Here's how the part is built. I have some questions about the finished solid (model axes, mm). Face numbers are marked on the shaded views. A direction names the side the tool comes from. Coordinates: 2 decimals unless noted, no trailing zeros. Order: outer loops, then holes, each group sorted by start corner. A loop starts at its lowest first (then second) coordinate and runs counter-clockwise, first axis right, second up. Notation, with made-up numbers: (13, 58) - (59, 58) arc R27 cw to (59, 80) - close; hole circle Ø4 at (65, 51). An arc over 180 degrees is marked (long way). Use one line per item in the form item = value. Start each with the question number.
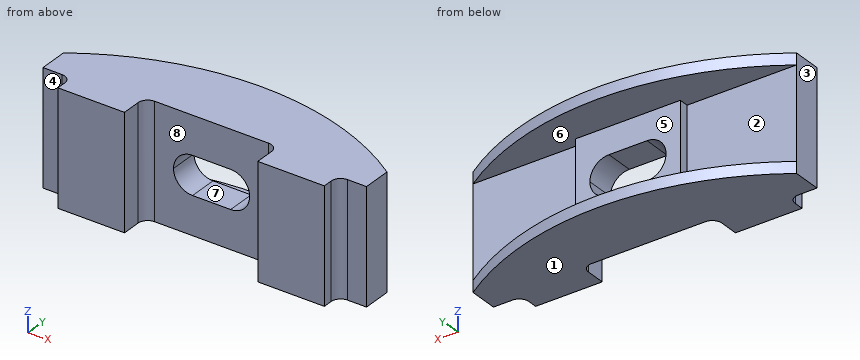
from build123d import *

# Parameters (mm, degrees)
F0_W      = 170
F0_H      = 60
F1_DEPTH  = 30
F2_W      = 70
F2_H      = 30
F3_DEPTH  = 59.69157
F4_R      = 5
F6_DEPTH  = 60.001
F7_W      = 57.5
F7_H      = 5
F8_DEPTH  = 60.001
F10_DEPTH = 6
F13_DEPTH = 30.001


with BuildPart() as f1:
    # F0 (on Front) → F1 (new body)
    with BuildSketch(Plane.XZ):
        Rectangle(F0_W, F0_H)
    extrude(amount=F1_DEPTH)

    # F2 (on Top) → F3 (cut, symmetric)
    with BuildSketch(Plane.XY):
        with Locations((0, -30)):
            Rectangle(F2_W, F2_H)
    extrude(amount=F3_DEPTH, both=True, mode=Mode.SUBTRACT)

    # F4
    f4_edges = [f1.edges().sort_by_distance(p)[0] for p in [
        (35, -15, 0),
        (-35, -15, 0),
    ]]
    fillet(f4_edges, radius=F4_R)

    # F5 (on face) → F6 (cut, through all)
    with BuildSketch(Plane.XY.offset(30)):
        with BuildLine():
            Line((70, -30), (85, -30))
            Line((85, -30), (85, -20))
            Line((85, -20), (75, -20))
            ThreePointArc((75, -20), (71.4644660941, -21.4644660941), (70, -25))
            Line((70, -25), (70, -30))
        make_face()
        with BuildLine():
            Line((-85, -20), (-85, -30))
            Line((-85, -30), (-70, -30))
            Line((-70, -30), (-70, -25))
            ThreePointArc((-70, -25), (-71.4644660941, -21.4644660941), (-75, -20))
            Line((-75, -20), (-85, -20))
        make_face()
    extrude(amount=-F6_DEPTH, mode=Mode.SUBTRACT)

    # F7 (on face) → F8 (cut, through all)
    with BuildSketch(Plane.XY.offset(30)):
        with Locations((56.25, -2.5)):
            Rectangle(F7_W, F7_H)
        with Locations((-56.25, -2.5)):
            Rectangle(F7_W, F7_H)
    extrude(amount=-F8_DEPTH, mode=Mode.SUBTRACT)

    # F9 (on face) → F10 (join)
    with BuildSketch(Plane.XY.offset(30)):
        with BuildLine():
            Line((27.5, -5), (85, -5))
            ThreePointArc((85, -5), (0, 21.4079290569), (-85, -5))
            Line((-85, -5), (-27.5, -5))
            Line((-27.5, -5), (-27.5, 0))
            Line((-27.5, 0), (27.5, 0))
            Line((27.5, 0), (27.5, -5))
        make_face()
    extrude(amount=-F10_DEPTH)

    # F11: F1 across plane


with BuildPart() as f1_1:
    add(f1.part)
    add(f1.part.mirror(Plane.XY))

    # F12 (on face) → F13 (cut, through all)
    with BuildSketch(Plane(origin=(0, 0, 0), x_dir=(-1, 0, 0), z_dir=(0, 1, 0))):
        with BuildLine():
            ThreePointArc((20, 0), (17.0710678119, 7.0710678119), (10, 10))
            Line((10, 10), (-10, 10))
            ThreePointArc((-10, 10), (-17.0710678119, 7.0710678119), (-20, 0))
            ThreePointArc((-20, 0), (-17.0710678119, -7.0710678119), (-10, -10))
            Line((-10, -10), (10, -10))
            ThreePointArc((10, -10), (17.0710678119, -7.0710678119), (20, 0))
        make_face()
    extrude(amount=-F13_DEPTH, mode=Mode.SUBTRACT)


solid = f1_1.part
1) I need wall thicknesses on probe 1 along Z at (x, y) = (-19.5, 8); probe 2 along X at (y, z) = (-26, -11); probe 3 along Z at (x, y) = (-5, -11). Which ranges of each line are inside material? Lowest first, please. Write a range as [from, to].
2) Which directions (+Z, -Z, +X, -X, +Y, -Y) give clear straight access to the entire face, cutting with the end or side of a thin tool? Please do the marked faces 4, 5, 6, 7 and 8.
3) For pin 1 (11 mm diameter, centred on y = -26, z = -4, fed in from -X); pin 2 (2.5 mm diameter, centred on y = -27, z = 12.5, fed in from +X); pin 3 (24 mm diameter, centred on x = -70, z = 2.5, fed in from +Y); pin 4 (18 mm diameter, centred on x = -8, z = 0, fed in from -Y), each with a flat end and sliding along its axis, tell me the tip position at first contact or that it passes through.
4) Suppose I cut it at A-A, the plane y = -9.5. List the corners of the cut face in (x, z) for me, then the cut area to 3 significant figures.
5) Suppose I cut it at D-D, the plane x = -40. List the corners of the cut face in (y, z) for me, then the cut area to 3 significant figures.
6) Suppose I cut it at C-C, the plane y = 7.5. List the corners of the cut face in (x, z) for me, then the cut area to 3 significant figures.
7) If we mould it in two halves opening along Z, with no side actions, what happens to the marked faces 1, 2 and 3? For each: pulls with the +Z half, pulls with the -Z half, needs draft (parallel to the pull), parting line crosses it, or undercut.
8) Suppose I cut it at B-B, the plane z = -8. List the corners of the cut face in (x, y) for me, then the cut area to 3 significant figures.
From the geometry:
q1.probe_1 = [-30, -24], [24, 30]
q1.probe_2 = [-70, -35], [35, 70]
q1.probe_3 = [-30, -10], [10, 30]
q2.face_4 = +Z, -Z, -X, -Y
q2.face_5 = +X, -X, +Y
q2.face_6 = +Y
q2.face_7 = +Y, -Y
q2.face_8 = +Z, -Z, -Y
q3.pin_1 = -72.82
q3.pin_2 = 70
q3.pin_3 = -5
q3.pin_4 = through
q4.outline = (-85, -30) - (85, -30) - (85, 30) - (-85, 30) - close; hole (-10, -10) - (10, -10) arc R10 ccw to (10, 10) - (-10, 10) arc R10 ccw to start
q4.area = 9,490 mm2
q5.outline = (-30, -30) - (15.98, -30) - (15.98, -24) - (-5, -24) - (-5, 24) - (15.98, 24) - (15.98, 30) - (-30, 30) - close
q5.area = 1,750 mm2
q6.outline = (-63.08, -30) - (63.08, -30) - (63.08, -24) - (-63.08, -24) - close; (-63.08, 24) - (63.08, 24) - (63.08, 30) - (-63.08, 30) - close
q6.area = 1,510 mm2
q7.face_1 = pulls with the -Z half
q7.face_2 = undercut
q7.face_3 = needs draft
q8.outline = (-85, -20) - (-75, -20) arc R5 cw to (-70, -25) - (-70, -30) - (-35, -30) - (-35, -20) arc R5 cw to (-30, -15) - (-16, -15) - (-16, 0) - (-27.5, 0) - (-27.5, -5) - (-85, -5) - close; (16, -15) - (30, -15) arc R5 cw to (35, -20) - (35, -30) - (70, -30) - (70, -25) arc R5 cw to (75, -20) - (85, -20) - (85, -5) - (27.5, -5) - (27.5, 0) - (16, 0) - close
q8.area = 2,720 mm2
